Autodesk Inventor part; units mm, degrees
ref_plane "YZ Plane" through (0, 0, 0) normal (1, 0, 0) x (0, 1, 0)
ref_plane "XZ Plane" through (0, 0, 0) normal (0, 1, 0) x (-1, 0, 0)
ref_plane "XY Plane" through (0, 0, 0) normal (0, 0, 1) x (1, 0, 0)
sketch "Sketch1" plane through (0, 0, 0) normal (0, 0, 1) x (1, 0, 0)
  arc A0 (-28.9184, -1.6435) -> (-32.3684, 5.7551) centre (-35.052, 0) ccw
  line L0 (-28.702, 47.5942) -> (-28.702, -124.4009) construction
  line L1 (-32.3684, 5.7551) -> (-88.9, 32.1162)
  line L2 (-28.9184, -1.6435) -> (-86.2301, -215.5338)
  line L3 (-46.4564, 12.3244) -> (-66.802, 12.3244)
  line L4 (-60.4508, -95.6256) -> (-54.1008, -95.6256)
  line L5 (-73.152, -5.9838) -> (-73.152, -131.1779)
  line L6 (-73.152, -131.1779) -> (-63.627, -131.1779)
  line L7 (58.5667, 38.1) -> (-194.088, 38.1) construction
  line L8 (-95.25, 6.7162) -> (-95.25, -5.9838)
  line L9 (-95.25, 6.7162) -> (-88.9, 6.7162)
  line L10 (-88.9, 6.7162) -> (-88.9, 32.1162)
  line L11 (-95.25, -5.9838) -> (-73.152, -5.9838)
  line L12 (-95.25, -5.9838) -> (-95.25, -18.6838)
  line L13 (-95.25, -18.6838) -> (-89.3064, -18.6838)
  line L14 (-89.3064, -18.6838) -> (-89.3064, -24.6274)
  line L15 (-89.3064, -24.6274) -> (-95.25, -24.6274)
  line L16 (-95.25, -24.6274) -> (-95.25, -82.1838)
  line L17 (-95.25, -82.1838) -> (-82.55, -82.1838)
  line L18 (-89.3064, -18.6838) -> (-82.55, -18.6838)
  line L19 (-82.55, -18.6838) -> (-82.55, -82.1838)
  line L20 (-95.25, -82.1838) -> (-101.6, -82.1838)
  line L21 (-66.802, 12.3244) -> (-66.802, -31.3838)
  line L22 (-66.802, -31.3838) -> (-60.4508, -95.6256)
  line L23 (-82.55, -178.1009) -> (-76.2, -178.1009)
  line L24 (-82.55, -82.1838) -> (-82.55, -178.1009)
  line L25 (-86.2301, -215.5338) -> (-89.4051, -215.5338)
  line L26 (-89.4051, -215.5338) -> (-101.6, -82.1838)
  line L27 (-69.977, -5.9838) -> (-69.977, -31.3838)
  line L28 (-69.977, -31.3838) -> (-73.152, -31.3838)
  line L29 (-69.977, -5.9838) -> (-66.802, -5.9838)
  line L30 (-101.6, -82.1838) -> (-28.702, -82.1838) construction
  line L31 (0, -268.1594) -> (0, 100.2199)
  point P0 (0, 0)
  dimension "d0" = 12.7
  dimension "d1" = 28.702
  dimension "d3" = 15
  dimension "d4" = 6.35
  dimension "d9" = 38.1
  dimension "d11" = 12.7
  dimension "d13" = 95.25
  dimension "d14" = 6.35
  dimension "d15" = 25.4
  dimension "d17" = 12.7
  dimension "d18" = 5.9436
  dimension "d19" = 5.9436
  dimension "d20" = 12.7
  dimension "d22" = 107.95
  dimension "d23" = 63.5
  dimension "d25" = 25.4
  dimension "d26" = 6.35
  dimension "d27" = 133.35
  dimension "d28" = 3.175
  dimension "d29" = 101.6
  dimension "d30" = 6.35
  dimension "d31" = 25
  dimension "d32" = 44.45
  dimension "d33" = 3.175
  dimension "d34" = 20.3456
  dimension "d35" = 9.525
revolve "Revolution1" add sketch "Sketch1" angle 360 about axis through (0, -10, 0) along (0, 1, 0) contours L2 L4 L22 L21 L3 L1 A0
properties part number "graphite" material "GFRC"
Work out the finished part from the listing and answer in its coordinate system (mm). Coordinates: 2 decimals unless noted, no trailing zeros. Write each loop counter-clockwise with the first axis right and the second up, starting at its lowest first coordinate (ties: lowest second). Pieces come first, ordered by that corner, then holes. Notation, with made-up numbers: M 49.25,68.5 L 78.25,68.5 A28 ccw 78.25,91.5 Z; hole C 66,40 d9. An arc over 180 degrees is marked long. Answer as CSV lines item,"result". Start each with the question number.
Item 1: Section C-C on y = -29.5 is taken. Write down the section's boundary in (x, z).
Item 2: Section A-A on z = 0 is taken. Write down the section's boundary in (x, y), and give its area (3 significant figures).
Item 3: Determine the mould class of faces 1 (the face through (14.481, -9.836, 65.213)), 2 (the face through (-14, 12.324, 45)), 3 (the face through (7.208, 6.166, -32.459)) for opening direction Z: released by +Z, released by -Z, zero draft, split by the parting line, or undercut.
Item 4: Section D-D on y = -16 is taken. Write down the section's boundary in (x, z), and give its area (3 significant figures).
Item 5: Flat-ended cylindrical pins translate along their axes: P1, Ø6, axis at x = 16, z = -18.5, coming from the -Y side; P2, Ø4, axis at x = 15, y = -20.5, coming from the -Z side; P3, Ø4, axis at x = -19.5, y = -37.5, coming from the -Z side; P4, Ø4, axis at y = 0, z = -27.5, coming from the -X side. Find the tip coordinate at first contact, or state that the pin passes through.
Item 6: Consider L1, parallel to Z at x = 44.5, y = -87; L2, parallel to X at y = -36.5, z = -7; L3, parallel to X at y = -65.5, z = 9. Determine where each line is inside the solid, lowest interval first.
Item 7: Section B-B on x = 0 is taken. Write down the section's boundary in (y, z), and give its area (3 significant figures).
Checks:
1,outline,"C 0,0 d133.6; hole C 0,0 d72.77"
2,outline,"M -66.8,-31.38 L -60.45,-95.63 L -54.1,-95.63 L -28.92,-1.64 A6.35 ccw -32.37,5.76 L -46.46,12.32 L -66.8,12.32 Z; M 28.92,-1.64 L 54.1,-95.63 L 60.45,-95.63 L 66.8,-31.38 L 66.8,12.32 L 46.46,12.32 L 32.37,5.76 A6.35 ccw Z"
2,area,"5,260 mm²"
3,face 1,"split by the parting line"
3,face 2,"zero draft"
3,face 3,"undercut"
4,outline,"C 0,0 d133.6; hole C 0,0 d65.53"
4,area,"10,600 mm²"
5,P1,"passes through"
5,P2,"stops at z = -65.52"
5,P3,"stops at z = -63.88"
5,P4,"stops at x = -61.74"
6,L1,"z = -42.16 to -26.49, 26.49 to 42.16"
6,L2,"x = -65.93 to -37.61, 37.61 to 65.93"
6,L3,"x = -62.79 to -45.14, 45.14 to 62.79"
7,outline,"M -95.63,-60.45 L -31.38,-66.8 L 12.32,-66.8 L 12.32,-46.46 L 5.76,-32.37 A6.35 ccw -1.64,-28.92 L -95.63,-54.1 Z; M -95.63,54.1 L -1.64,28.92 A6.35 ccw 5.76,32.37 L 12.32,46.46 L 12.32,66.8 L -31.38,66.8 L -95.63,60.45 Z"
7,area,"5,260 mm²"
